Check sheet for the modelled part. Datum: model origin and axes. Units: mm. A direction names the side the tool comes from. Give positions to 0.01 mm unless a question says otherwise; leave off trailing zeros. Order: outer loops, then holes, each group sorted by start corner. A loop starts at its lowest first (then second) coordinate and runs counter-clockwise, first axis right, second up. Notation, with made-up numbers: M -27.5,34.5 L -4.5,34.5 A20 cw -4.5,60.5 Z; hole C 50,-17.5 d6. An arc over 180 degrees is marked long. Return JSON: item names as keys, results as strings. Group by question number.
Autodesk Fusion 360 part; units mm, degrees
sketch "スケッチ1" plane through (0, 0, 0) normal (0, 1, 0) x (1, 0, 0)
  line L0 (-100, 0) -> (100, 0) construction
  line L1 (0, 100) -> (0, -100) construction
  line L2 (-40, 40) -> (40, 40)
  line L3 (40, 40) -> (40, -40)
  line L4 (40, -40) -> (-40, -40)
  line L5 (-40, -40) -> (-40, 40)
  line L6 (-40, 8) -> (-15, 8)
  line L7 (-15, 8) -> (-15, -8)
  line L8 (-15, -8) -> (-40, -8)
  line L9 (-40, -8) -> (-40, 8)
  circle A0 centre (-35, 0) radius 2.25
  circle A1 centre (-20, 0) radius 2.25
  circle A2 centre (0, 0) radius 35 construction
  circle A3 centre (0, 0) radius 40 construction
  circle A4 centre (-35, 35) radius 1.25
  circle A5 centre (35, 35) radius 1.25
  circle A6 centre (-35, -35) radius 1.25
  circle A7 centre (35, -35) radius 1.25
  circle A8 centre (-35, 0) radius 4.25
  circle A9 centre (-20, 0) radius 4.25
  line L10 (-50, 50) -> (50, 50)
  line L11 (50, 50) -> (50, -50)
  line L12 (50, -50) -> (-50, -50)
  line L13 (-50, -50) -> (-50, 50)
  line L14 (-48, 48) -> (48, 48)
  line L15 (48, 48) -> (48, -48)
  line L16 (48, -48) -> (-48, -48)
  line L17 (-48, -48) -> (-48, 48)
  dimension "d1" = 40
  dimension "d2" = 40
  dimension "d3" = 40
  dimension "d4" = 40
  dimension "d5" = 4.5
  dimension "d6" = 4.5
  dimension "d7" = 15
  dimension "d8" = 5
  dimension "d9" = 25
  dimension "d10" = 8
  dimension "d11" = 8
  dimension "d12" = 70
  dimension "d13" = 80
  dimension "d14" = 2.5
  dimension "d15" = 2.5
  dimension "d16" = 2.5
  dimension "d17" = 2.5
  dimension "d18" = 5
  dimension "d19" = 5
  dimension "d20" = 5
  dimension "d21" = 5
  dimension "d22" = 5
  dimension "d23" = 5
  dimension "d24" = 5
  dimension "d25" = 5
  dimension "d26" = 8.5
  dimension "d27" = 8.5
  dimension "d35" = 50
  dimension "d36" = 50
  dimension "d37" = 50
  dimension "d38" = 50
  dimension "d39" = 2
  dimension "d40" = 2
  dimension "d41" = 2
  dimension "d42" = 2
extrude "押し出し1" add sketch "スケッチ1" against normal blind 3 contours L2 L3 L4 L5 L6 L7 L8 | L14 L15 L16 L17
extrude "押し出し2" add sketch "スケッチ1" against normal blind 8 contours L5 L6 L7 L8 L9
extrude "押し出し3" add sketch "スケッチ1" against normal blind 4 from surface at -4 contours A8 | A9
fillet "フィレット1" radius 2 2 edges at (-38.9624, -4, -1.5369) (-23.9624, -4, -1.5369)
extrude "押し出し4" add sketch "スケッチ1" against normal blind 15 contours L10 L11 L12 L13
sketch "スケッチ2" plane through (0, 0, 0) normal (0, 0, 1) x (1, 0, 0)
fillet "フィレット2" radius 3 8 edges at (48, -9, 48) (48, -9, -48) (-48, -9, -48) (-48, -9, 48) (0, -3, -48) (48, -3, 0) (0, -3, 48) (-48, -3, 0)
fillet "フィレット3" radius 5 8 edges at (0, 0, -50) (50, -7.5, -50) (50, 0, 0) (50, -7.5, 50) (0, 0, 50) (-50, 0, 0) (-50, -7.5, 50) (-50, -7.5, -50)
1) Material ranges on line 1 along X through (y, z) = (-7, 0); line 2 along X through (y, z) = (-7.75, 7); line 3 along X through (y, z) = (-6, 15), recorded low to high.
2) Depth check by flat-ended pin: P1, Ø2, axis at x = -33.5, y = -3.5, coming from the +Z side; P2, Ø5, axis at x = -36, z = -1, coming from the +Y side; P3, Ø1.5, axis at x = -35, z = -35, coming from the -Y side; P4, Ø5, axis at x = -27, z = 0, coming from the -Y side. Enter the tip coordinate at first touch or a pass-through.
3) Sectioned sample at B-B on z = 35. Record the boundary of the cut face in (x, y), then the cut area to 3 significant figures.
4) Tool access check on faces 1 (the face through (-17.854, -5.972, -0.676)), 2 (the face through (-47.14, -10.56, -47.1)). Record the directions out of +Z, -Z, +X, -X, +Y, -Y that give a thin tool (end or side, any length) a straight path to the whole face; none if there is none.
5) Sectioned sample at C-C on y = -12. Record the boundary of the cut face in (x, z).
6) Release check for a two-part mould opening along Z. For faces 3 (the face through (-48.4, -15, -22.5)), 4 (the face through (34.73, -1.48, -33.78)), 5 (the face through (48, -10, -49)), 6 (the face through (-28, -5, -8)) record: released by +Z, released by -Z, zero draft, split by the parting line, or undercut.
7) Sectioned sample at A-A on x = 35. Record the boundary of the cut face in (y, z).
Reply:
{
 "1": {"line 1": "-50 to -48, -40 to -37.25, -32.75 to -22.25, -17.75 to -15, 48 to 50", "line 2": "-50 to -48, -40 to -15, 48 to 50", "line 3": "-50 to -48, 48 to 50"},
 "2": {"P1": "z = 49.97", "P2": "y = -3.11", "P3": "through", "P4": "y = -8"},
 "3": {"outline": "M -50,-15 L -48,-15 L -48,-6 A3 cw -45,-3 L -36.25,-3 L -36.25,0 L -45,0 A5 ccw -50,-5 Z; M -33.75,-3 L 33.75,-3 L 33.75,0 L -33.75,0 Z; M 36.25,-3 L 45,-3 A3 cw 48,-6 L 48,-15 L 50,-15 L 50,-5 A5 ccw 45,0 L 36.25,0 Z", "area": "326 mm^2"},
 "4": {"face 1": "+Y, -Y", "face 2": "-Y"},
 "5": {"outline": "M -50,-45 A5 ccw -45,-50 L 45,-50 A5 ccw 50,-45 L 50,45 A5 ccw 45,50 L -45,50 A5 ccw -50,45 Z; hole M -48,-45 A3 ccw -45,-48 L 45,-48 A3 ccw 48,-45 L 48,45 A3 ccw 45,48 L -45,48 A3 ccw -48,45 Z"},
 "6": {"face 3": "zero draft", "face 4": "undercut", "face 5": "released by -Z", "face 6": "undercut"},
 "7": {"outline": "M -15,-50 L -5,-50 A5 ccw 0,-45 L 0,-36.25 L -3,-36.25 L -3,-45 A3 cw -6,-48 L -15,-48 Z; M -15,48 L -6,48 A3 cw -3,45 L -3,36.25 L 0,36.25 L 0,45 A5 ccw -5,50 L -15,50 Z; M -3,-33.75 L 0,-33.75 L 0,33.75 L -3,33.75 Z"}
}
